Autodesk Inventor part; units mm, degrees
ref_plane "YZ Plane" through (0, 0, 0) normal (1, 0, 0) x (0, 1, 0)
ref_plane "XZ Plane" through (0, 0, 0) normal (0, 1, 0) x (-1, 0, 0)
ref_plane "XY Plane" through (0, 0, 0) normal (0, 0, 1) x (1, 0, 0)
sketch "Sketch1" plane through (0, 0, 0) normal (0, 1, 0) x (-1, 0, 0)
  line L0 (0, 0) -> (25.4, 0)
  line L1 (25.4, 0) -> (25.4, -25.4)
  line L2 (25.4, -25.4) -> (0, -25.4)
  line L3 (0, -25.4) -> (0, 0)
  line L4 (22.225, -3.175) -> (3.175, -3.175)
  line L5 (3.175, -3.175) -> (3.175, -22.225)
  line L6 (3.175, -22.225) -> (22.225, -22.225)
  line L7 (22.225, -22.225) -> (22.225, -3.175)
  line L8 (22.225, -3.175) -> (25.4, -3.175)
  line L9 (3.175, -22.225) -> (3.175, -25.4)
  dimension "d0" = 25.4
  dimension "d1" = 25.4
  dimension "d2" = 3.175
extrude "Extrusion1" add sketch "Sketch1" along normal blind 228.6 contours L0 L1 L8 L4 L5 L9 L2 L3
properties part number "BumberGussetFront.ver1-1111-2020"
Could you check a few things on this model? Use its own coordinates, in mm. A direction names the side the tool comes from. Give positions to 0.01 mm unless a question says otherwise; leave off trailing zeros. Order: outer loops, then holes, each group sorted by start corner. A loop starts at its lowest first (then second) coordinate and runs counter-clockwise, first axis right, second up. Notation, with made-up numbers: (-21, 15) -> (37, 15) arc R38 ccw to (37, 54) -> close; hole circle Ø10 at (-25.5, 23.5). An arc over 180 degrees is marked (long way). Answer in a Markdown table with one row per item. Add a question column.
Item 1: I'm going to push flat-ended pins straight in: P1, Ø10, axis at x = -18, y = 201.5, coming from the -Z side (3 decimals); P2, Ø2, axis at y = 78.5, z = -13.5, coming from the -X side (3 decimals). Where does each tip first touch, or does it pass through?
Item 2: Imagine slicing it at A-A (y = 129.5). List the corners of the cut face in (x, z) for me (3 decimals).
Item 3: Please list where this line runs through material, in increasing order: probe 1 along Z at (x, y) = (-11.25, 154.5) (3 decimals).
Item 4: For faces 1 (the flat face through (-2, 228.6, -7)), 2 (the flat face through (-3.175, 113, -14)), which set-ups out of +Z, -Z, +X, -X, +Y, -Y let a thin tool reach every point of the face, with its end or its side?
Item 5: Imagine slicing it at B-B (z = -15). List the corners of the cut face in (x, y) for me (3 decimals).
Item 6: Imagine slicing it at C-C (x = -16.5). List the corners of the cut face in (y, z) for me (3 decimals), and give its area (3 significant figures).
Result:
| question | item | result |
|---|---|---|
| 1 | P1 | z = -3.175 |
| 1 | P2 | x = -3.175 |
| 2 | outline | (-25.4, -3.175) -> (-3.175, -3.175) -> (-3.175, -25.4) -> (0, -25.4) -> (0, 0) -> (-25.4, 0) -> close |
| 3 | probe 1 | -3.175 to 0 |
| 4 | face 1 | +Z, -Z, +X, -X, +Y |
| 4 | face 2 | -Z, -X, +Y, -Y |
| 5 | outline | (-3.175, 0) -> (0, 0) -> (0, 228.6) -> (-3.175, 228.6) -> close |
| 6 | outline | (0, -3.175) -> (228.6, -3.175) -> (228.6, 0) -> (0, 0) -> close |
| 6 | area | 726 mm2 |
